Autodesk Inventor part; units mm, degrees
ref_plane "YZ Plane" through (0, 0, 0) normal (1, 0, 0) x (0, 1, 0)
ref_plane "XZ Plane" through (0, 0, 0) normal (0, 1, 0) x (-1, 0, 0)
ref_plane "XY Plane" through (0, 0, 0) normal (0, 0, 1) x (1, 0, 0)
sketch "Sketch1" plane through (0, 0, 0) normal (0, 1, 0) x (-1, 0, 0)
  line L0 (23, -50) -> (-23, -50)
  line L1 (-23, -50) -> (-23, 50)
  line L2 (-23, 50) -> (23, 50)
  line L3 (23, 50) -> (23, -50)
  line L4 (0, -70) -> (0, 70)
  line L5 (-32.2, 0) -> (32.2, 0)
  point P0 (0, 0)
  dimension "d0" = 46
  dimension "d1" = 100
extrude "Extrusion1" add sketch "Sketch1" along normal blind 2
fillet "Fillet1" radius 2.5 4 edges at (-23, 1, -50) (-23, 1, 50) (23, 1, -50) (23, 1, 50)
sketch "Sketch6" plane through (0, 0, 0) normal (0, -1, 0) x (1, 0, 0)
  line L0 (21.5, -42.7) -> (17, -42.7)
  line L1 (17, -42.7) -> (17, -20.7)
  line L2 (17, -20.7) -> (21.5, -20.7)
  line L3 (21.5, -20.7) -> (21.5, -42.7)
  line L4 (20.5, -50) -> (-20.5, -50)
  line L5 (23, 47.5) -> (23, -47.5)
  line L6 (0, 70) -> (0, -70)
  line L7 (-32.2, 0) -> (32.2, 0)
  line L8 (-21.5, -42.7) -> (-17, -42.7)
  line L9 (-17, -42.7) -> (-17, -20.7)
  line L10 (-17, -20.7) -> (-21.5, -20.7)
  line L11 (-21.5, -20.7) -> (-21.5, -42.7)
  line L12 (21.5, 42.7) -> (17, 42.7)
  line L13 (17, 42.7) -> (17, 20.7)
  line L14 (17, 20.7) -> (21.5, 20.7)
  line L15 (21.5, 20.7) -> (21.5, 42.7)
  line L16 (-21.5, 42.7) -> (-17, 42.7)
  line L17 (-17, 42.7) -> (-17, 20.7)
  line L18 (-17, 20.7) -> (-21.5, 20.7)
  line L19 (-21.5, 20.7) -> (-21.5, 42.7)
  point P0 (0, 0)
  dimension "d50" = 4.5
  dimension "d51" = 22
  dimension "d52" = 7.3
  dimension "d53" = 1.5
extrude "Extrusion6" cut sketch "Sketch6" against normal through all
sketch "Sketch7" plane through (0, 0, 0) normal (0, -1, 0) x (1, 0, 0)
  line L0 (17, -20.7) -> (21.5, -20.7)
  line L1 (19.5, 17.35) -> (19.5, -17.35)
  line L2 (20.35, -17.35) -> (20.35, 17.35)
  line L3 (23, 47.5) -> (23, -47.5)
  line L4 (0, 70) -> (0, -70)
  line L5 (-32.2, 0) -> (32.2, 0)
  line L6 (21.5, 20.7) -> (17, 20.7)
  line L7 (15.35, 47.35) -> (-15.35, 47.35)
  line L8 (-15.35, 46.5) -> (15.35, 46.5)
  line L9 (-20.5, 50) -> (20.5, 50)
  line L10 (-15.371, 47.35) -> (-15.35, 47.35)
  line L11 (20.35, 17.35) -> (19.5, 17.35)
  line L12 (20.35, -17.35) -> (19.5, -17.35)
  line L13 (15.35, 46.5) -> (15.35, 47.35)
  line L14 (17, 20.7) -> (17, 42.7)
  line L15 (-15.35, 46.5) -> (-15.35, 47.35)
  line L16 (-17, 42.7) -> (-17, 20.7)
  line L17 (15.35, -47.35) -> (-15.35, -47.35)
  line L18 (-15.35, -46.5) -> (15.35, -46.5)
  line L19 (-15.371, -47.35) -> (-15.35, -47.35)
  line L20 (15.35, -46.5) -> (15.35, -47.35)
  line L21 (-15.35, -46.5) -> (-15.35, -47.35)
  line L22 (-17, -20.7) -> (-21.5, -20.7)
  line L23 (-19.5, 17.35) -> (-19.5, -17.35)
  line L24 (-20.35, -17.35) -> (-20.35, 17.35)
  line L25 (-21.5, 20.7) -> (-17, 20.7)
  line L26 (-20.35, 17.35) -> (-19.5, 17.35)
  line L27 (-20.35, -17.35) -> (-19.5, -17.35)
  line L28 (-23, -47.5) -> (-23, 47.5)
  point P0 (0, 0)
  dimension "d57" = 3.5
  dimension "d65" = 3.5
  dimension "d67" = 3.35
  dimension "d68" = 0.85
  dimension "d69" = 3.35
  dimension "d70" = 0.85
  dimension "d75" = 7.65
  dimension "d76" = 7.65
extrude "Extrusion7" add sketch "Sketch7" along normal blind 5
properties part number "horni1"
Read the model definition and answer for the solid it produces. Units are mm, in the model's axes. A direction names the side the tool comes from. Give positions to 0.01 mm unless a question says otherwise; leave off trailing zeros. Write each loop counter-clockwise with the first axis right and the second up, starting at its lowest first coordinate (ties: lowest second). Pieces come first, ordered by that corner, then holes. Notation, with made-up numbers: (25.5, 13) -> (82.5, 13) arc R17 cw to (82.5, 38) -> close; hole circle Ø8 at (89.5, 53). An arc over 180 degrees is marked (long way). Answer as a JSON object with one key per item and string values.
1) Flat-ended cylindrical pins translate along their axes: pin 1 Ø2.5 at (y, z) = (-1.5, 1) entering from -X; pin 2 Ø2.5 at (x, y) = (0, -2) entering from -Z; pin 3 Ø0.7 at (y, z) = (-3.5, -47) entering from -X. Find the tip coordinate at first contact, or state that the pin passes through.
Findings below:
{"pin 1": "stops at x = -20.35", "pin 2": "stops at z = -47.35", "pin 3": "stops at x = -15.35"}
2) Section B-B on y = -1 is taken. Write down the section's boundary in (x, z), then the cut area to 3 significant figures.
Findings below:
{"outline": "(-20.35, -17.35) -> (-19.5, -17.35) -> (-19.5, 17.35) -> (-20.35, 17.35) -> close; (-15.35, -47.35) -> (15.35, -47.35) -> (15.35, -46.5) -> (-15.35, -46.5) -> close; (-15.35, 46.5) -> (15.35, 46.5) -> (15.35, 47.35) -> (-15.35, 47.35) -> close; (19.5, -17.35) -> (20.35, -17.35) -> (20.35, 17.35) -> (19.5, 17.35) -> close", "area": "111 mm^2"}
3) A tool of negligible diameter and unlimited length cuts with its end or side. For faces 1 (the flat face through (0, -2, 47.35)), 2 (the flat face through (0, -2, 46.5)), 3 (the flat face through (20.35, -2, 0)), 4 (the flat face through (-19.5, -2, 0)), 5 (the flat face through (19, 1, 42.7)), from which of +Z, -Z, +X, -X, +Y, -Y can it reach the whole face along a straight path? Write none if from no direction.
Findings below:
{"face 1": "+Z, +X, -X, -Y", "face 2": "+X, -X, -Y", "face 3": "+Z, -Z, +X, -Y", "face 4": "+Z, -Z, -Y", "face 5": "+Y, -Y"}
4) Section C-C on x = 2.5 is taken. Write down the section's boundary in (y, z), then the cut area to 4 significant figures.
Findings below:
{"outline": "(-5, -47.35) -> (0, -47.35) -> (0, -50) -> (2, -50) -> (2, 50) -> (0, 50) -> (0, 47.35) -> (-5, 47.35) -> (-5, 46.5) -> (0, 46.5) -> (0, -46.5) -> (-5, -46.5) -> close", "area": "208.5 mm^2"}
5) Straight lines are drawn through the part: probe 1 along X at (y, z) = (0.5, 41); probe 2 along Z at (x, y) = (-20, 1.5); probe 3 along Z at (x, y) = (-2, -3.5). For each, find the intervals that lie inside material, in ascending order. Write a range as from..to.
Findings below:
{"probe 1": "x = -23..-21.5, -17..17, 21.5..23", "probe 2": "z = -50..-42.7, -20.7..20.7, 42.7..50", "probe 3": "z = -47.35..-46.5, 46.5..47.35"}
6) Section D-D on z = -13 is taken. Write down the section's boundary in (x, y).
Findings below:
{"outline": "(-23, 0) -> (-20.35, 0) -> (-20.35, -5) -> (-19.5, -5) -> (-19.5, 0) -> (19.5, 0) -> (19.5, -5) -> (20.35, -5) -> (20.35, 0) -> (23, 0) -> (23, 2) -> (-23, 2) -> close"}
7) Section A-A on z = 35.5 is taken. Write down the section's boundary in (x, y).
Findings below:
{"outline": "(-23, 0) -> (-21.5, 0) -> (-21.5, 2) -> (-23, 2) -> close; (-17, 0) -> (17, 0) -> (17, 2) -> (-17, 2) -> close; (21.5, 0) -> (23, 0) -> (23, 2) -> (21.5, 2) -> close"}
